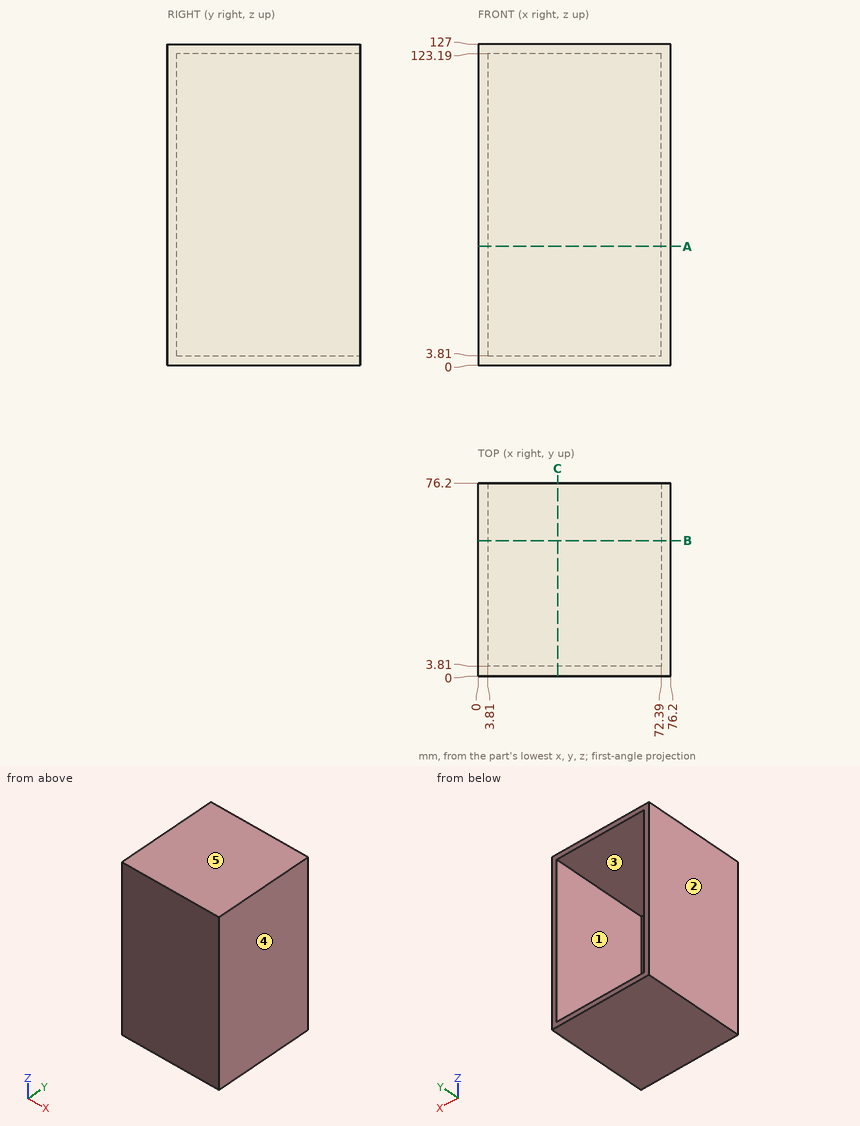
Study the drawing (mm; zero at the part's minimum x, y, z) and answer. A direction names the side the tool comes from. Give positions to 0.01 mm unless a question says otherwise; leave off trailing zeros. Write each loop counter-clockwise with the first axis right and the second up, starting at its lowest first coordinate (ties: lowest second). Pieces come first, ordered by that corner, then holes. Notation, with made-up numbers: (-35.75, 42) -> (-28.75, 42) arc R8 cw to (-28.75, 51) -> close; hole circle Ø3 at (27.5, 16). An arc over 180 degrees is marked (long way). Answer as a JSON object with one key per item and string values. Group by question number.
1) Find section C-C (x = 31.5). Write down the section's boundary in (y, z).
2) Find section A-A (z = 47). Write down the section's boundary in (x, y).
3) Find section B-B (y = 53.5). Write down the section's boundary in (x, z), and give its area (3 significant figures).
4) Consider L1, parallel to X at y = 6, z = 86; L2, parallel to Z at x = 62, y = 42; L3, parallel to Y at x = 18, z = 32. Determine where each line is inside the solid, lowest interval first. Write a range as from..to.
5) A tool of negligible diameter and unlimited length cuts with its end or side. For the marked faces 1 and 2, from which of +Z, -Z, +X, -X, +Y, -Y can it reach the whole face along a straight path? Write none if from no direction.
6) This flat-tipped pin is pushed along its axis until it touches: P1, Ø1, axis at y = 41, z = 43, coming from the -X side. Where does it stop, or does it pass through?
7) The mould has two halves that part along Z. Classify the marked faces 3, 4 and 5: +Z half, -Z half, draft (parallel to the pull), parting line (faces both ways), or undercut.
Values follow:
{
 "1": {"outline": "(0, 0) -> (76.2, 0) -> (76.2, 3.81) -> (3.81, 3.81) -> (3.81, 123.19) -> (76.2, 123.19) -> (76.2, 127) -> (0, 127) -> close"},
 "2": {"outline": "(0, 0) -> (76.2, 0) -> (76.2, 76.2) -> (72.39, 76.2) -> (72.39, 3.81) -> (3.81, 3.81) -> (3.81, 76.2) -> (0, 76.2) -> close"},
 "3": {"outline": "(0, 0) -> (76.2, 0) -> (76.2, 127) -> (0, 127) -> close; hole (3.81, 3.81) -> (72.39, 3.81) -> (72.39, 123.19) -> (3.81, 123.19) -> close", "area": "1,490 mm2"},
 "4": {"L1": "x = 0..3.81, 72.39..76.2", "L2": "z = 0..3.81, 123.19..127", "L3": "y = 0..3.81"},
 "5": {"face 1": "+Y", "face 2": "+Z, -Z, -X, +Y, -Y"},
 "6": {"P1": "stops at x = 0"},
 "7": {"face 3": "undercut", "face 4": "draft", "face 5": "+Z half"}
}
